Can you work these out from the drawing? Everything is in mm from the part's minimum corner. Round coordinates to 2 decimals unless told otherwise and drop trailing zeros. Order: outer loops, then holes, each group sorted by start corner. A loop starts at its lowest first (then second) coordinate and runs counter-clockwise, first axis right, second up. Notation, with made-up numbers: M 53,49.5 L 78,49.5 A18 ccw 78,80.5 Z; hole C -29,73 d6. An arc over 180 degrees is marked long. Write each question's results on one line, items separated by ' | '. Start each with the question number.
1. Suppose I cut it at C-C on y = 20. Write out the boundary of the cut face in (x, z).
2. Please list where these lines run through material, in increasing order: L1, parallel to X at y = 2, z = 0.3; L2, parallel to X at y = 19, z = 2.95; L3, parallel to Y at x = 32.5, z = 2.65.
3. I'm going to push flat-ended pins straight in: pin 1 (0.9 mm diameter, centred on y = 36, z = 2, fed in from -X); pin 2 (1.5 mm diameter, centred on y = 2, z = 1, fed in from +X); pin 3 (1.6 mm diameter, centred on x = 1.5, z = 1, fed in from -Y). Where does each tip first touch, or does it pass through?
4. Suppose I cut it at B-B on x = 18.5. Write out the boundary of the cut face in (y, z).
5. Suppose I cut it at A-A on y = 4. Write out the boundary of the cut face in (x, z), and give its area (3 significant figures).
6. Suppose I cut it at D-D on z = 1.1. Give the number of separate pieces and of enclosed holes in the cut face, and give its area (3 significant figures).
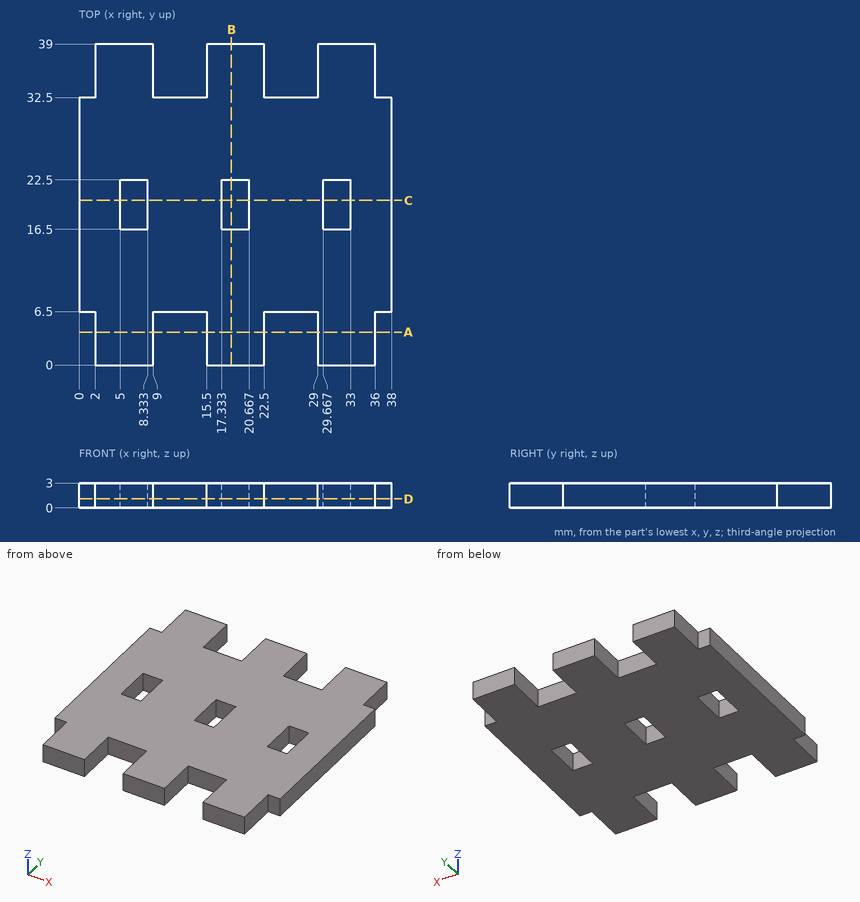
Filled sheet:
1) outline: M 0,0 L 5,0 L 5,3 L 0,3 Z; M 8.33,0 L 17.33,0 L 17.33,3 L 8.33,3 Z; M 20.67,0 L 29.67,0 L 29.67,3 L 20.67,3 Z; M 33,0 L 38,0 L 38,3 L 33,3 Z
2) L1: x = 2 to 9, 15.5 to 22.5, 29 to 36 | L2: x = 0 to 5, 8.33 to 17.33, 20.67 to 29.67, 33 to 38 | L3: y = 0 to 16.5, 22.5 to 39
3) pin 1: stops at x = 2 | pin 2: stops at x = 36 | pin 3: stops at y = 0
4) outline: M 0,0 L 16.5,0 L 16.5,3 L 0,3 Z; M 22.5,0 L 39,0 L 39,3 L 22.5,3 Z
5) outline: M 2,0 L 9,0 L 9,3 L 2,3 Z; M 15.5,0 L 22.5,0 L 22.5,3 L 15.5,3 Z; M 29,0 L 36,0 L 36,3 L 29,3 Z | area: 63.0 mm^2
6) separate pieces: 1 | enclosed holes: 3 | area: 1,200 mm^2
